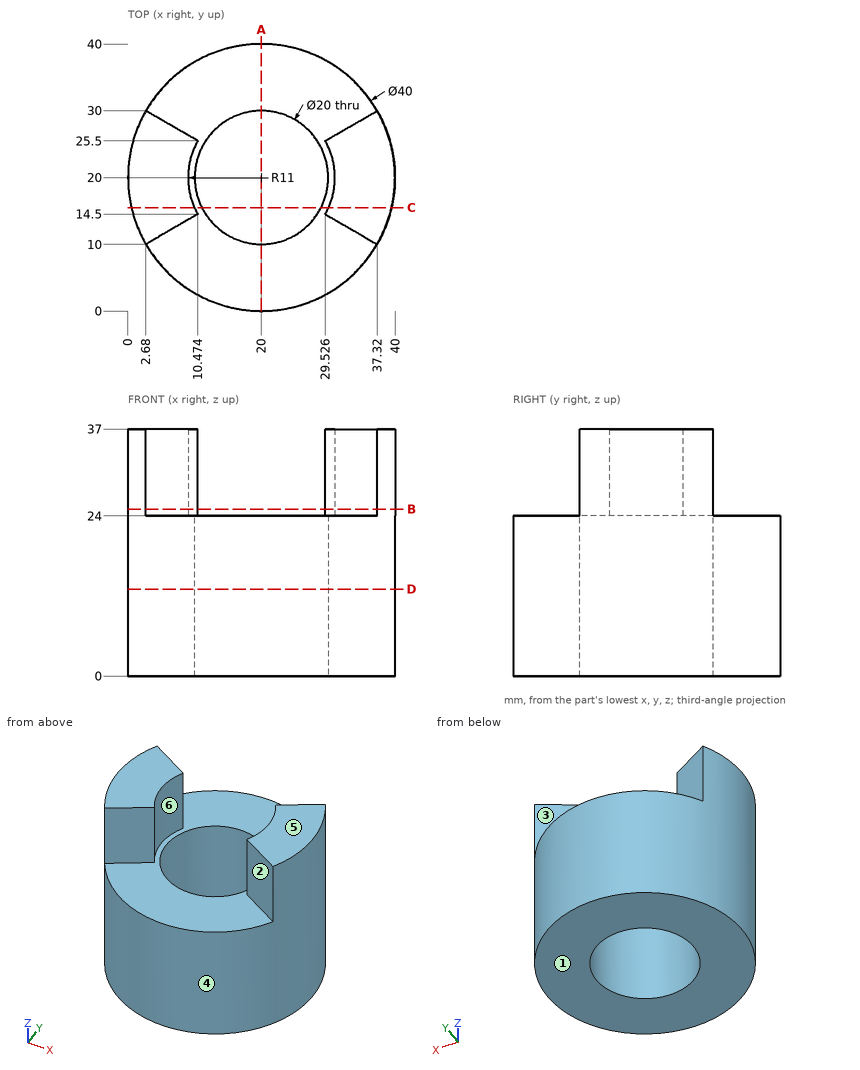
Part print with two shaded views. Sizes in mm from the minimum x, y, z corner. A direction names the side the tool comes from. Round coordinates to 2 decimals unless told otherwise and drop trailing zeros. Order: outer loops, then holes, each group sorted by start corner. A loop starts at its lowest first (then second) coordinate and runs counter-clockwise, first axis right, second up. Notation, with made-up numbers: (0.5, -36.75) -> (34.5, -36.75) arc R26 cw to (34.5, -0.75) -> close; hole circle Ø4 at (-26.75, -36). An arc over 180 degrees is marked (long way). One line per question, with ' | ' between items.
Q1. Which spindle directions (+Z, -Z, +X, -X, +Y, -Y) get a long thin tool onto all of the face, cutting with end or side? Do the marked faces 1, 2 and 3. Say none if no direction does.
Completed:
face 1: -Z, +X, -X, +Y, -Y | face 2: +Z, -Y | face 3: +Z, +Y
Q2. Slice it at C-C (y = 15.5). Write the cut outline in (x, z).
Completed:
outline: (0.51, 0) -> (11.07, 0) -> (11.07, 24) -> (9.96, 24) -> (9.96, 37) -> (0.51, 37) -> close; (28.93, 0) -> (39.49, 0) -> (39.49, 37) -> (30.04, 37) -> (30.04, 24) -> (28.93, 24) -> close
Q3. Probe probe 1 along Y at (x, z) = (20, 10); probe 2 along Z at (x, y) = (16, 7); probe 3 along Y at (x, z) = (21.5, 18.5). List the from-to ranges inside material, lowest first.
Completed:
probe 1: y = 0 to 10, 30 to 40 | probe 2: z = 0 to 24 | probe 3: y = 0.06 to 10.11, 29.89 to 39.94
Q4. Two-plate mould, pull along X, no slides. Class the marked faces 4, 5 and 6: released by +X, released by -X, zero draft, split by the parting line, or undercut.
Completed:
face 4: split by the parting line | face 5: zero draft | face 6: undercut
Q5. Slice it at D-D (z = 13). Write the cut outline in (x, y).
Completed:
outline: circle Ø40 at (20, 20); hole circle Ø20 at (20, 20)
Q6. Slice it at B-B (z = 25). Write the cut outline in (x, y).
Completed:
outline: (2.68, 10) -> (10.47, 14.5) arc R11 cw to (10.47, 25.5) -> (2.68, 30) arc R20 ccw to start; (29.53, 14.5) -> (37.32, 10) arc R20 ccw to (37.32, 30) -> (29.53, 25.5) arc R11 cw to start
Q7. Slice it at A-A (x = 20). Write the cut outline in (y, z), then the cut area to 3 significant figures.
Completed:
outline: (0, 0) -> (10, 0) -> (10, 24) -> (0, 24) -> close; (30, 0) -> (40, 0) -> (40, 24) -> (30, 24) -> close | area: 480 mm^2
Q8. Drop flat-ended pins along their axis: pin 1 (12 mm diameter, centred on x = 8, z = 17.5, fed in from -Y); pin 2 (6 mm diameter, centred on y = 23.5, z = 31, fed in from -X); pin 3 (10 mm diameter, centred on x = 14, z = 13, fed in from +Y) (1 decimal); pin 4 (12 mm diameter, centred on x = 20, y = 20, fed in from +Z). Give the stop position or say it passes through.
Completed:
pin 1: stops at y = 0.92 | pin 2: stops at x = 0.01 | pin 3: stops at y = 40 | pin 4: passes through
